Source: CAD feature listing. Evaluate the final solid. Frame: model axes, mm. A direction names the side the tool comes from. Round coordinates to 2 decimals unless told otherwise and drop trailing zeros. Write each loop counter-clockwise with the first axis right and the second up, starting at its lowest first coordinate (ties: lowest second). Pieces come first, ordered by that corner, then holes. Notation, with made-up numbers: M -4.75,1.5 L 23.25,1.5 A21 ccw 23.25,17.5 Z; hole C 37.5,36 d8. An arc over 180 degrees is marked long. Use a Markdown table: item, result.
Autodesk Inventor part; units mm, degrees
ref_plane "YZ Plane" through (0, 0, 0) normal (1, 0, 0) x (0, 1, 0)
ref_plane "XZ Plane" through (0, 0, 0) normal (0, 1, 0) x (-1, 0, 0)
ref_plane "XY Plane" through (0, 0, 0) normal (0, 0, 1) x (1, 0, 0)
sketch "Sketch1" plane through (0, 0, 0) normal (0, 0, 1) x (1, 0, 0)
  line L0 (0, 0) -> (115, 0)
  line L1 (115, 0) -> (115, 75)
  line L2 (115, 75) -> (0, 75)
  line L3 (0, 75) -> (0, 0)
  dimension "d0" = 115
  dimension "d1" = 75
extrude "Extrusion1" add sketch "Sketch1" along normal blind 40
sketch "Sketch2" plane through (0, 0, 40) normal (0, 0, 1) x (1, 0, 0)
  line L0 (115, 75) -> (0, 75)
  line L1 (115, 0) -> (115, 75)
  line L2 (0, 75) -> (115, 75)
  line L3 (115, 75) -> (115, 55)
  line L4 (115, 55) -> (0, 55)
  line L5 (0, 55) -> (0, 75)
  point P0 (0, 0)
  dimension "d4" = 20
extrude "Extrusion2" cut sketch "Sketch2" against normal blind 5
sketch "Sketch3" plane through (115, 0, 0) normal (1, 0, 0) x (0, 0, -1)
  line L0 (0, 75) -> (-35, 75)
  line L1 (-35, 75) -> (-35, 55)
  line L2 (-35, 55) -> (-40, 55)
  line L3 (-40, 0) -> (-40, 55)
  line L4 (0, 0) -> (-40, 0)
  line L5 (0, 70) -> (-30, 70)
  line L6 (-30, 70) -> (-30, 50)
  line L7 (-30, 50) -> (-35, 50)
  line L8 (-35, 50) -> (-35, 5)
  line L9 (-35, 5) -> (0, 5)
  line L10 (0, 5) -> (0, 70)
  line L11 (0, 0) -> (0, 75)
  dimension "d7" = 5
extrude "Extrusion3" cut sketch "Sketch3" against normal through all contours L10 L9 L8 L7 L6 L5
sketch "Sketch4" plane through (115, 5, 35) normal (0, 0, -1) x (-1, 0, 0)
  line L0 (0, 45) -> (115, 45)
  line L1 (115, 0) -> (0, 0)
  line L2 (115, 45) -> (110, 45)
  line L3 (110, 45) -> (110, 0)
  line L4 (110, 0) -> (115, 0)
  line L5 (115, 0) -> (115, 45)
  point P0 (115, -5)
  dimension "d10" = 5
extrude "Extrusion4" add sketch "Sketch4" along normal blind 5
sketch "Sketch5" plane through (115, 50, 30) normal (0, 0, -1) x (-1, 0, 0)
  line L0 (115, 20) -> (115, -45)
  line L1 (115, -45) -> (110, -45)
  line L2 (110, -45) -> (110, 0)
  line L3 (110, 0) -> (115, 0)
  line L4 (115, 0) -> (115, -45)
  point P0 (115, -50)
  dimension "d13" = 5
  dimension "d14" = 45
extrude "Extrusion5" add sketch "Sketch5" along normal blind 30
sketch "Sketch6" plane through (0, 0, 0) normal (0, 0, -1) x (-1, 0, 0)
  line L0 (-5, 5) -> (-5, 50)
  line L1 (-5, 5) -> (-50, 5)
  line L2 (-50, 5) -> (-50, 50)
  line L3 (-50, 50) -> (-5, 50)
  line L4 (-5, 50) -> (-5, 5)
  point P0 (0, 0)
  dimension "d17" = 45
  dimension "d18" = 45
extrude "Extrusion6" add sketch "Sketch6" against normal blind 5
sketch "Sketch7" plane through (0, 0, 0) normal (0, 0, -1) x (-1, 0, 0)
  line L0 (0, 50) -> (-50, 50) construction
  line L1 (-5, 5) -> (-5, 50) construction
  line L2 (-50, 50) -> (-5, 50) construction
  line L3 (-5, 50) -> (-5, 5) construction
  line L4 (-5, 5) -> (-50, 5) construction
  line L5 (-50, 5) -> (-50, 50) construction
  line L6 (-43, 12) -> (-12, 12) construction
  line L7 (-12, 12) -> (-12, 43) construction
  line L8 (-12, 43) -> (-43, 43) construction
  line L9 (-43, 43) -> (-43, 12) construction
  line L10 (-43, 12) -> (-12, 43) construction
  line L11 (-12, 12) -> (-43, 43) construction
  circle A0 centre (-43, 43) radius 1.5
  circle A1 centre (-12, 43) radius 1.5
  circle A2 centre (-43, 12) radius 1.5
  circle A3 centre (-12, 12) radius 1.5
  circle A4 centre (-27.5, 27.5) radius 3
  point P0 (0, 0)
  point P1 (-50, 27.5)
  point P2 (-27.5, 50)
  dimension "d21" = 45
  dimension "d22" = 45
  dimension "d23" = 31
  dimension "d24" = 31
  dimension "d25" = 3
  dimension "d26" = 3
  dimension "d27" = 3
  dimension "d28" = 3
  dimension "d29" = 6
extrude "Extrusion7" cut sketch "Sketch7" against normal blind 5
sketch "Sketch8" plane through (0, 0, 0) normal (0, 0, -1) x (-1, 0, 0)
  circle A0 centre (-27.5, 27.5) radius 3
  circle A1 centre (-27.5, 27.5) radius 12.5
  point P0 (0, 0)
  dimension "d32" = 25
extrude "Extrusion8" cut sketch "Sketch8" against normal blind 2
sketch "Sketch9" plane through (115, 50, 30) normal (0, 0, -1) x (-1, 0, 0)
  line L0 (115, 5) -> (115, -50)
  line L1 (115, 0) -> (65, 0)
  line L2 (65, 0) -> (65, 5)
  line L3 (65, 5) -> (115, 5)
  line L4 (115, 5) -> (115, 0)
  dimension "d35" = 50
  dimension "d36" = 5
extrude "Extrusion9" add sketch "Sketch9" along normal blind 30
sketch "Sketch10" plane through (115, 5, 35) normal (0, 0, -1) x (-1, 0, 0)
  circle A0 centre (87.5, 22.5) radius 3
  circle A1 centre (87.5, 22.5) radius 12.5
  point P0 (115, -5)
  dimension "d39" = 25
extrude "Extrusion10" add sketch "Sketch10" along normal blind 5 contours A0 | A1
sketch "Sketch11" plane through (0, 0, 0) normal (0, 0, -1) x (-1, 0, 0)
  line L0 (-120, 70) -> (5, 70)
  line L1 (5, 70) -> (5, 65)
  line L2 (5, 65) -> (-120, 65)
  line L3 (-120, 65) -> (-120, 70)
  line L4 (-115, 70) -> (-115, 75)
  point P0 (0, 0)
  point P1 (0, 70)
  dimension "d42" = 5
  dimension "d43" = 5
  dimension "d44" = 5
extrude "Extrusion11" add sketch "Sketch11" against normal blind 30
properties part number "FA003" material "ABS Plastic"
Q1. Section D-D on y = 27.5. Return loops of the section in (x, z), plus the area to 3 significant figures.
Results are:
| item | result |
|---|---|
| outline | M 0,0 L 15,0 L 15,2 L 24.5,2 L 24.5,5 L 5,5 L 5,35 L 15,35 L 15,30 L 40,30 L 40,35 L 115,35 L 115,40 L 0,40 Z; M 30.5,2 L 40,2 L 40,0 L 50,0 L 50,5 L 30.5,5 Z |
| area | 1,030 mm^2 |
Q2. Reachability of faces 1 (the cylindrical face through (13.5, 12.07, 2.46)), 2 (the flat face through (58, 75, 17)), 3 (the flat face through (57, 0, 20)), 4 (the flat face through (61, 5, 18)), 5 (the flat face through (57, 65, 15)) from +Z, -Z, +X, -X, +Y, -Y: full face, straight path, thin tool, end or side. Return the list, or none.
Results are:
| item | result |
|---|---|
| face 1 | -Z |
| face 2 | +Z, -Z, +X, -X, +Y |
| face 3 | +Z, -Z, +X, -X, -Y |
| face 4 | +X |
| face 5 | -Z, +X, -X |
Q3. Section A-A on x = 43. Return loops of the section in (y, z).
Results are:
| item | result |
|---|---|
| outline | M 0,0 L 10.5,0 L 10.5,5 L 5,5 L 5,35 L 50,35 L 50,5 L 44.5,5 L 44.5,0 L 55,0 L 55,30 L 65,30 L 65,0 L 75,0 L 75,35 L 55,35 L 55,40 L 0,40 Z; M 13.5,0 L 41.5,0 L 41.5,5 L 13.5,5 Z |
Q4. First-contact query: pin 1 Ø2.5 at (x, y) = (-3, 66.5) entering from +Z; pin 2 Ø7.5 at (x, y) = (24.5, 33.5) entering from -Z; pin 3 Ø1 at (x, z) = (64.5, 30.5) entering from -Y; pin 4 Ø1.8 at (x, y) = (43, 43) entering from -Z. Flat tips, straight axial feed; report the tip coordinate or a pass-through.
Results are:
| item | result |
|---|---|
| pin 1 | z = 30 |
| pin 2 | z = 2 |
| pin 3 | y = 0 |
| pin 4 | z = 35 |
Q5. Line query: L1, parallel to Y at x = 43, z = 2; L2, parallel to Y at x = 27.5, z = 4.35; L3, parallel to Z at x = 21.5, y = 40. Output: solid intervals per line, ascending.
Results are:
| item | result |
|---|---|
| L1 | 0 to 10.5, 13.5 to 41.5, 44.5 to 55, 65 to 75 |
| L2 | 0 to 24.5, 30.5 to 55, 65 to 75 |
| L3 | 0 to 5, 35 to 40 |
Q6. Section C-C on z = 7. Return loops of the section in (x, y), plus the area to 3 significant figures.
Results are:
| item | result |
|---|---|
| outline | M -5,65 L 120,65 L 120,70 L 115,70 L 115,75 L 0,75 L 0,70 L -5,70 Z; M 0,0 L 115,0 L 115,5 L 5,5 L 5,50 L 50,50 L 50,55 L 0,55 Z |
| area | 2,250 mm^2 |
Q7. Mould query, pull axis X, two halves, no side actions, for faces 6 (the flat face through (-2, 68, 30)), 7 (the cylindrical face through (37.42, 19.894, 0.986)), 8 (the flat face through (-5, 68, 15)), 9 (the flat face through (50, 39, 4)). Classes: +X half, -X half, draft (parallel to the pull), parting line (faces both ways), or undercut.
Results are:
| item | result |
|---|---|
| face 6 | draft |
| face 7 | undercut |
| face 8 | -X half |
| face 9 | +X half |
Q8. Section B-B on y = 12. Return loops of the section in (x, z), plus the area to 3 significant figures.
Results are:
| item | result |
|---|---|
| outline | M 0,0 L 10.5,0 L 10.5,5 L 5,5 L 5,35 L 115,35 L 115,40 L 0,40 Z; M 13.5,0 L 41.5,0 L 41.5,5 L 13.5,5 Z; M 44.5,0 L 50,0 L 50,5 L 44.5,5 Z |
| area | 945 mm^2 |
